Model file for the job. Use its own axes, mm. Round coordinates to 2 decimals unless told otherwise and drop trailing zeros. Order: outer loops, then holes, each group sorted by start corner. A loop starts at its lowest first (then second) coordinate and runs counter-clockwise, first axis right, second up. Notation, with made-up numbers: (79.25, 32) - (107.25, 32) arc R27 cw to (107.25, 57) - close; hole circle Ø6 at (61, 79). An arc over 180 degrees is marked (long way). Write item = value, one per line. Start each with the question number.
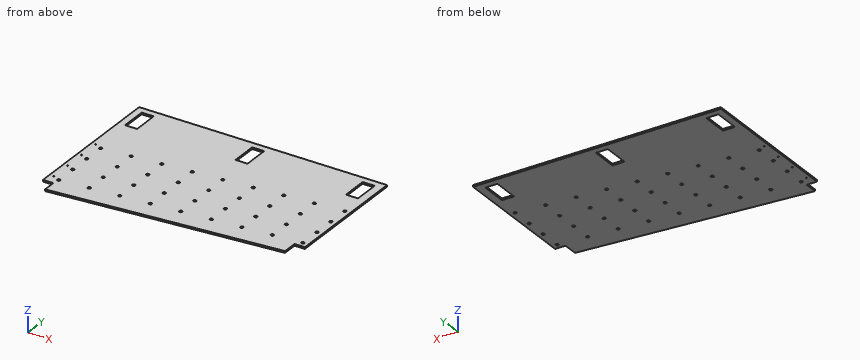
Autodesk Fusion 360 part; units mm, degrees
sketch "Sketch1" plane through (0, 0, 0) normal (0, 0, 1) x (1, 0, 0)
  line L0 (0, 0) -> (914.4, 0)
  line L1 (914.4, 0) -> (914.4, 600.8)
  line L2 (914.4, 600.8) -> (0, 600.8)
  line L3 (0, 600.8) -> (0, 0)
  dimension "d1" = 914.4
  dimension "d2" = 600.8
extrude "Extrude1" add sketch "Sketch1" along normal blind 6.35
sketch "Sketch4" plane through (0, 0, 6.35) normal (0, 0, 1) x (1, 0, 0)
  circle A0 centre (894.4, 150.8) radius 5.3675
  line L0 (0, 0) -> (800, 0)
  line L1 (914.4, 0) -> (914.4, 600.8)
  line L2 (0, 600.8) -> (0, 0)
  line L3 (0, 0) -> (914.4, 0)
  line L4 (914.4, 0) -> (914.4, 600.8)
  line L5 (914.4, 600.8) -> (0, 600.8)
  dimension "d6" = 10.735
  dimension "d8" = 150.8
  dimension "d38" = 20
extrude "Extrude2" cut sketch "Sketch4" against normal blind 35 contours A0
sketch "Sketch5" plane through (0, 0, 6.35) normal (0, 0, 1) x (1, 0, 0)
  circle A0 centre (894.4, 150.8) radius 5.3675
  line L0 (0, 600.8) -> (0, 0)
  line L1 (0, 0) -> (914.4, 0)
  line L2 (914.4, 0) -> (914.4, 600.8)
  line L3 (914.4, 600.8) -> (0, 600.8)
  line L4 (894.4, 150.8) -> (97.4442, 81.0754)
  line L5 (894.4, 150.8) -> (1694.4, 150.8) construction
  dimension "d11" = 175
  dimension "d12" = 800
pattern_linear "R-Pattern1" count 9 spacing 107 along (-0.9962, -0.0872, 0) count 4 spacing 80 along (0, 1, 0) of "Extrude2"
sketch "Sketch6" plane through (0, 0, 6.35) normal (0, 0, 1) x (1, 0, 0)
  circle A0 centre (41.6573, 316.1947) radius 5.3675
  circle A1 centre (148.2502, 325.5203) radius 5.3675
  circle A2 centre (254.843, 334.846) radius 5.3675
  circle A3 centre (361.4358, 344.1717) radius 5.3675
  circle A4 centre (468.0287, 353.4973) radius 5.3675
  circle A5 centre (574.6215, 362.823) radius 5.3675
  circle A6 centre (681.2143, 372.1487) radius 5.3675
  circle A7 centre (787.8072, 381.4743) radius 5.3675
  circle A8 centre (894.4, 390.8) radius 5.3675
  circle A9 centre (41.6573, 236.1947) radius 5.3675
  circle A10 centre (148.2502, 245.5203) radius 5.3675
  circle A11 centre (254.843, 254.846) radius 5.3675
  circle A12 centre (361.4358, 264.1717) radius 5.3675
  circle A13 centre (468.0287, 273.4973) radius 5.3675
  circle A14 centre (574.6215, 282.823) radius 5.3675
  circle A15 centre (681.2143, 292.1487) radius 5.3675
  circle A16 centre (787.8072, 301.4743) radius 5.3675
  circle A17 centre (894.4, 310.8) radius 5.3675
  circle A18 centre (41.6573, 156.1947) radius 5.3675
  circle A19 centre (148.2502, 165.5203) radius 5.3675
  circle A20 centre (254.843, 174.846) radius 5.3675
  circle A21 centre (361.4358, 184.1717) radius 5.3675
  circle A22 centre (468.0287, 193.4973) radius 5.3675
  circle A23 centre (574.6215, 202.823) radius 5.3675
  circle A24 centre (681.2143, 212.1487) radius 5.3675
  circle A25 centre (787.8072, 221.4743) radius 5.3675
  circle A26 centre (894.4, 230.8) radius 5.3675
  circle A27 centre (41.6573, 76.1947) radius 5.3675
  circle A28 centre (148.2502, 85.5203) radius 5.3675
  circle A29 centre (254.843, 94.846) radius 5.3675
  circle A30 centre (361.4358, 104.1717) radius 5.3675
  circle A31 centre (468.0287, 113.4973) radius 5.3675
  circle A32 centre (574.6215, 122.823) radius 5.3675
  circle A33 centre (681.2143, 132.1487) radius 5.3675
  circle A34 centre (787.8072, 141.4743) radius 5.3675
  circle A35 centre (894.4, 150.8) radius 5.3675
  line L0 (0, 600.8) -> (0, 0)
  line L1 (0, 0) -> (914.4, 0)
  line L2 (914.4, 0) -> (914.4, 600.8)
  line L3 (914.4, 600.8) -> (0, 600.8)
  line L4 (69.85, 576.0244) -> (69.85, 480.7744)
  line L5 (69.85, 480.7744) -> (25.4, 480.7744)
  line L6 (25.4, 480.7744) -> (25.4, 576.024)
  line L7 (25.4, 576.024) -> (69.85, 576.0244)
  line L8 (0, 600.8) -> (0, 0)
  line L9 (914.4, 600.8) -> (0, 600.8)
  line L10 (0, 0) -> (800, 0)
  dimension "d17" = 95.25
  dimension "d18" = 44.45
  dimension "d39" = 25.4
  dimension "d42" = 44.45
  dimension "d43" = 480.7744
extrude "Extrude3" cut sketch "Sketch6" against normal blind 100 contours L4 L5 L6 L7
pattern_linear "R-Pattern2" count 3 spacing 407.5 along (1, 0, 0) of "Extrude3"
sketch "Sketch7" plane through (0, 0, 6.35) normal (0, 0, 1) x (1, 0, 0)
  line L0 (884.85, 480.7744) -> (840.4, 480.7744)
  line L1 (840.4, 480.7744) -> (840.4, 576.024)
  line L2 (840.4, 576.024) -> (884.85, 576.0244)
  line L3 (884.85, 576.0244) -> (884.85, 480.7744)
  line L4 (477.35, 480.7744) -> (432.9, 480.7744)
  line L5 (432.9, 480.7744) -> (432.9, 576.024)
  line L6 (432.9, 576.024) -> (477.35, 576.0244)
  line L7 (477.35, 576.0244) -> (477.35, 480.7744)
  line L8 (69.85, 480.7744) -> (25.4, 480.7744)
  line L9 (25.4, 480.7744) -> (25.4, 576.024)
  line L10 (25.4, 576.024) -> (69.85, 576.0244)
  line L11 (69.85, 576.0244) -> (69.85, 480.7744)
  circle A0 centre (41.6573, 316.1947) radius 5.3675
  circle A1 centre (148.2502, 325.5203) radius 5.3675
  circle A2 centre (254.843, 334.846) radius 5.3675
  circle A3 centre (361.4358, 344.1717) radius 5.3675
  circle A4 centre (468.0287, 353.4973) radius 5.3675
  circle A5 centre (574.6215, 362.823) radius 5.3675
  circle A6 centre (681.2143, 372.1487) radius 5.3675
  circle A7 centre (787.8072, 381.4743) radius 5.3675
  circle A8 centre (894.4, 390.8) radius 5.3675
  circle A9 centre (41.6573, 236.1947) radius 5.3675
  circle A10 centre (148.2502, 245.5203) radius 5.3675
  circle A11 centre (254.843, 254.846) radius 5.3675
  circle A12 centre (361.4358, 264.1717) radius 5.3675
  circle A13 centre (468.0287, 273.4973) radius 5.3675
  circle A14 centre (574.6215, 282.823) radius 5.3675
  circle A15 centre (681.2143, 292.1487) radius 5.3675
  circle A16 centre (787.8072, 301.4743) radius 5.3675
  circle A17 centre (894.4, 310.8) radius 5.3675
  circle A18 centre (41.6573, 156.1947) radius 5.3675
  circle A19 centre (148.2502, 165.5203) radius 5.3675
  circle A20 centre (254.843, 174.846) radius 5.3675
  circle A21 centre (361.4358, 184.1717) radius 5.3675
  circle A22 centre (468.0287, 193.4973) radius 5.3675
  circle A23 centre (574.6215, 202.823) radius 5.3675
  circle A24 centre (681.2143, 212.1487) radius 5.3675
  circle A25 centre (787.8072, 221.4743) radius 5.3675
  circle A26 centre (894.4, 230.8) radius 5.3675
  circle A27 centre (41.6573, 76.1947) radius 5.3675
  circle A28 centre (148.2502, 85.5203) radius 5.3675
  circle A29 centre (254.843, 94.846) radius 5.3675
  circle A30 centre (361.4358, 104.1717) radius 5.3675
  circle A31 centre (468.0287, 113.4973) radius 5.3675
  circle A32 centre (574.6215, 122.823) radius 5.3675
  circle A33 centre (681.2143, 132.1487) radius 5.3675
  circle A34 centre (787.8072, 141.4743) radius 5.3675
  circle A35 centre (894.4, 150.8) radius 5.3675
  line L12 (0, 600.8) -> (0, 0)
  line L13 (0, 0) -> (914.4, 0)
  line L14 (914.4, 0) -> (914.4, 600.8)
  line L15 (914.4, 600.8) -> (0, 600.8)
  line L16 (0, 0) -> (914.4, 79.9996)
  line L17 (0, 0) -> (803.0559, 0) construction
  line L18 (914.4, 79.9996) -> (914.4, 0)
  line L19 (914.4, 0) -> (0, 0)
  dimension "d25" = 5
extrude "Extrude4" cut sketch "Sketch7" against normal blind 150 contours L13 L14 L16 L18 L19
sketch "Sketch8" plane through (0, 0, 6.35) normal (0, 0, 1) x (1, 0, 0)
  line L0 (0, 0) -> (914.4, 79.9996)
  line L1 (914.4, 79.9996) -> (914.4, 600.8)
  line L2 (914.4, 600.8) -> (0, 600.8)
  line L3 (0, 600.8) -> (0, 0)
  circle A0 centre (894.4, 150.8) radius 5.3675
  circle A1 centre (787.8072, 141.4743) radius 5.3675
  circle A2 centre (681.2143, 132.1487) radius 5.3675
  circle A3 centre (574.6215, 122.823) radius 5.3675
  circle A4 centre (468.0287, 113.4973) radius 5.3675
  circle A5 centre (361.4358, 104.1717) radius 5.3675
  circle A6 centre (254.843, 94.846) radius 5.3675
  circle A7 centre (148.2502, 85.5203) radius 5.3675
  circle A8 centre (41.6573, 76.1947) radius 5.3675
  circle A9 centre (894.4, 230.8) radius 5.3675
  circle A10 centre (787.8072, 221.4743) radius 5.3675
  circle A11 centre (681.2143, 212.1487) radius 5.3675
  circle A12 centre (574.6215, 202.823) radius 5.3675
  circle A13 centre (468.0287, 193.4973) radius 5.3675
  circle A14 centre (361.4358, 184.1717) radius 5.3675
  circle A15 centre (254.843, 174.846) radius 5.3675
  circle A16 centre (148.2502, 165.5203) radius 5.3675
  circle A17 centre (41.6573, 156.1947) radius 5.3675
  circle A18 centre (894.4, 310.8) radius 5.3675
  circle A19 centre (787.8072, 301.4743) radius 5.3675
  circle A20 centre (681.2143, 292.1487) radius 5.3675
  circle A21 centre (574.6215, 282.823) radius 5.3675
  circle A22 centre (468.0287, 273.4973) radius 5.3675
  circle A23 centre (361.4358, 264.1717) radius 5.3675
  circle A24 centre (254.843, 254.846) radius 5.3675
  circle A25 centre (148.2502, 245.5203) radius 5.3675
  circle A26 centre (41.6573, 236.1947) radius 5.3675
  circle A27 centre (894.4, 390.8) radius 5.3675
  circle A28 centre (787.8072, 381.4743) radius 5.3675
  circle A29 centre (681.2143, 372.1487) radius 5.3675
  circle A30 centre (574.6215, 362.823) radius 5.3675
  circle A31 centre (468.0287, 353.4973) radius 5.3675
  circle A32 centre (361.4358, 344.1717) radius 5.3675
  circle A33 centre (254.843, 334.846) radius 5.3675
  circle A34 centre (148.2502, 325.5203) radius 5.3675
  circle A35 centre (41.6573, 316.1947) radius 5.3675
  line L4 (69.85, 480.7744) -> (25.4, 480.7744)
  line L5 (25.4, 480.7744) -> (25.4, 576.024)
  line L6 (25.4, 576.024) -> (69.85, 576.0244)
  line L7 (69.85, 576.0244) -> (69.85, 480.7744)
  line L8 (477.35, 480.7744) -> (432.9, 480.7744)
  line L9 (432.9, 480.7744) -> (432.9, 576.024)
  line L10 (432.9, 576.024) -> (477.35, 576.0244)
  line L11 (477.35, 576.0244) -> (477.35, 480.7744)
  line L12 (884.85, 480.7744) -> (840.4, 480.7744)
  line L13 (840.4, 480.7744) -> (840.4, 576.024)
  line L14 (840.4, 576.024) -> (884.85, 576.0244)
  line L15 (884.85, 576.0244) -> (884.85, 480.7744)
  circle A36 centre (15, 88.3) radius 2.25
  dimension "d28" = 4.5
  dimension "d29" = 88.3
  dimension "d30" = 15
extrude "Extrude5" cut sketch "Sketch8" against normal blind 35 contours A36
pattern_linear "R-Pattern3" count 4 spacing 80 along (0, 1, 0) of "Extrude5"
sketch "Sketch9" plane through (0, 0, 6.35) normal (0, 0, 1) x (1, 0, 0)
  circle A0 centre (15, 328.3) radius 2.25
  circle A1 centre (15, 248.3) radius 2.25
  circle A2 centre (15, 168.3) radius 2.25
  circle A3 centre (15, 88.3) radius 2.25
  line L0 (0, 0) -> (914.4, 79.9996)
  line L1 (914.4, 79.9996) -> (914.4, 600.8)
  line L2 (914.4, 600.8) -> (0, 600.8)
  line L3 (0, 600.8) -> (0, 0)
  circle A4 centre (894.4, 150.8) radius 5.3675
  circle A5 centre (787.8072, 141.4743) radius 5.3675
  circle A6 centre (681.2143, 132.1487) radius 5.3675
  circle A7 centre (574.6215, 122.823) radius 5.3675
  circle A8 centre (468.0287, 113.4973) radius 5.3675
  circle A9 centre (361.4358, 104.1717) radius 5.3675
  circle A10 centre (254.843, 94.846) radius 5.3675
  circle A11 centre (148.2502, 85.5203) radius 5.3675
  circle A12 centre (41.6573, 76.1947) radius 5.3675
  circle A13 centre (894.4, 230.8) radius 5.3675
  circle A14 centre (787.8072, 221.4743) radius 5.3675
  circle A15 centre (681.2143, 212.1487) radius 5.3675
  circle A16 centre (574.6215, 202.823) radius 5.3675
  circle A17 centre (468.0287, 193.4973) radius 5.3675
  circle A18 centre (361.4358, 184.1717) radius 5.3675
  circle A19 centre (254.843, 174.846) radius 5.3675
  circle A20 centre (148.2502, 165.5203) radius 5.3675
  circle A21 centre (41.6573, 156.1947) radius 5.3675
  circle A22 centre (894.4, 310.8) radius 5.3675
  circle A23 centre (787.8072, 301.4743) radius 5.3675
  circle A24 centre (681.2143, 292.1487) radius 5.3675
  circle A25 centre (574.6215, 282.823) radius 5.3675
  circle A26 centre (468.0287, 273.4973) radius 5.3675
  circle A27 centre (361.4358, 264.1717) radius 5.3675
  circle A28 centre (254.843, 254.846) radius 5.3675
  circle A29 centre (148.2502, 245.5203) radius 5.3675
  circle A30 centre (41.6573, 236.1947) radius 5.3675
  circle A31 centre (894.4, 390.8) radius 5.3675
  circle A32 centre (787.8072, 381.4743) radius 5.3675
  circle A33 centre (681.2143, 372.1487) radius 5.3675
  circle A34 centre (574.6215, 362.823) radius 5.3675
  circle A35 centre (468.0287, 353.4973) radius 5.3675
  circle A36 centre (361.4358, 344.1717) radius 5.3675
  circle A37 centre (254.843, 334.846) radius 5.3675
  circle A38 centre (148.2502, 325.5203) radius 5.3675
  circle A39 centre (41.6573, 316.1947) radius 5.3675
  line L4 (69.85, 480.7744) -> (25.4, 480.7744)
  line L5 (25.4, 480.7744) -> (25.4, 576.024)
  line L6 (25.4, 576.024) -> (69.85, 576.0244)
  line L7 (69.85, 576.0244) -> (69.85, 480.7744)
  line L8 (477.35, 480.7744) -> (432.9, 480.7744)
  line L9 (432.9, 480.7744) -> (432.9, 576.024)
  line L10 (432.9, 576.024) -> (477.35, 576.0244)
  line L11 (477.35, 576.0244) -> (477.35, 480.7744)
  line L12 (884.85, 480.7744) -> (840.4, 480.7744)
  line L13 (840.4, 480.7744) -> (840.4, 576.024)
  line L14 (840.4, 576.024) -> (884.85, 576.0244)
  line L15 (884.85, 576.0244) -> (884.85, 480.7744)
  line L16 (0, 0) -> (38.1, 0)
  line L17 (38.1, 0) -> (38.1, 50.8)
  line L18 (38.1, 50.8) -> (0, 50.8)
  line L19 (0, 50.8) -> (0, 0)
  line L20 (876.3, 79.9996) -> (876.3, 130.7996)
  line L21 (876.3, 130.7996) -> (914.4, 130.7996)
  line L22 (914.4, 130.7996) -> (914.4, 79.9996)
  line L23 (876.3, 79.9996) -> (876.3, 76.6663)
  line L24 (914.4, 79.9996) -> (876.3, 76.6663)
  dimension "d44" = 38.1
  dimension "d45" = 50.8
  dimension "d46" = 38.1
  dimension "d47" = 50.8
extrude "Extrude6" cut sketch "Sketch9" against normal through all contours L0 L1 L20 L21 L22 L23 L24 | L0 L3 L17 L18 L19
equation "d2 = 550 mm + 2 in"
equation "d8 = 100 mm + 2 in"
equation "d29 = 37.5 mm + 2 in"
equation "d43 = 429.9744283331 mm + 2 in"
Item 1: Saw through at A-A, the plane x = 804. Give the cut face in (y, z).
Item 2: Drop flat-ended pins along their axis: pin 1 (2 mm diameter, centred on x = 207, y = 247.5, fed in from -Z); pin 2 (2 mm diameter, centred on x = 735.5, z = 5.5, fed in from -Y); pin 3 (3 mm diameter, centred on y = 114.5, z = 2, fed in from +X). Give the stop position or say it passes through.
Item 3: Saw through at C-C, the plane x = 378. Give the cut face in (y, z), then the cut area to 3 significant figures.
Item 4: Probe L1, parallel to X at y = 560, z = 4.5; L2, parallel to X at y = 168.3, z = 2; L3, parallel to X at y = 390.8, z = 3.25. List the from-to ranges inside material, lowest first.
Item 5: Saw through at B-B, the plane z = 5. Give the number of separate pieces and of enclosed holes in the cut face, then the cut area to 3 significant figures.
Check sheet entries:
q1.outline = (70.34, 0) - (600.8, 0) - (600.8, 6.35) - (70.34, 6.35) - close
q2.pin_1 = 0
q2.pin_2 = 64.26
q2.pin_3 = 876.3
q3.outline = (33.07, 0) - (600.8, 0) - (600.8, 6.35) - (33.07, 6.35) - close
q3.area = 3,610 mm2
q4.L1 = 0 to 25.4, 69.85 to 432.9, 477.35 to 840.4, 884.85 to 914.4
q4.L2 = 0 to 12.75, 17.25 to 143.66, 152.84 to 914.4
q4.L3 = 0 to 889.03, 899.77 to 914.4
q5.separate_pieces = 1
q5.enclosed_holes = 43
q5.area = 493,000 mm2
